from build123d import *

# Parameters (mm, degrees)
SKETCH1_W           = 38.1
SKETCH1_H           = 19.05
BOSS_EXTRUDE1_DEPTH = 12.7


with BuildPart() as part:
    # Sketch1 → Boss-Extrude1 (new body)
    with BuildSketch(Plane.XY):
        Rectangle(SKETCH1_W, SKETCH1_H)
    extrude(amount=BOSS_EXTRUDE1_DEPTH)

    # Sketch2 → Revolve1 (revolve)
    with BuildSketch(Plane(origin=(0, 0, 0), x_dir=(0, 0, -1), z_dir=(1, 0, 0))):
        Polygon((0, 0), (-800, 647.827226556), (-800, 0), align=None)
    revolve(axis=Axis((0, 0, 800), (0, 0, -1)))


solid = part.part
The model under review builds one solid part; all positions refer to its coordinate system, in mm. Give positions to 0.01 mm unless a question says otherwise; leave off trailing zeros. Loops run counter-clockwise (first coordinate to the right, second up) from the corner with the lowest first, then second, coordinate; pieces in that order, holes last. Notation, with made-up numbers: (-19.75, -38) -> (8.25, -38) arc R16 cw to (8.25, -11) -> close; hole circle Ø3 at (15.5, 22). An arc over 180 degrees is marked (long way). Answer as a JSON object with one key per item and string values. Group by question number.
Q1. Insertion check: pin 1 (1 mm diameter, centred on y = 50, z = 383, fed in from -X); pin 2 (2 mm diameter, centred on x = -401.5, z = 575.5, fed in from -Y); pin 3 (4 mm diameter, centred on y = 349, z = 692.5, fed in from -X). Each pin has a flat end and moves straight along its axis. Give the tip position at first contact, or say it passes through.
Q2. Take a section at B-B (z = 478). Write out the cut boundary in (x, y).
Q3. Wall thickness on line 1 along Y through (x, z) = (173, 371.5); line 2 along X through (y, z) = (-320, 680); line 3 along X through (y, z) = (7.5, 402.5): over which ranges is each line inside the solid? List them lowest first.
Q4. Take a section at A-A (z = 87). Write out the cut boundary in (x, y), plus the area to 3 significant figures.
Answer below:
{
 "1": {"pin 1": "stops at x = -306.51", "pin 2": "stops at y = -238.92", "pin 3": "stops at x = -441.54"},
 "2": {"outline": "circle Ø774.15 at (0, 0)"},
 "3": {"line 1": "y = -246.11 to 246.11", "line 2": "x = -448.13 to 448.13", "line 3": "x = -325.85 to 325.85"},
 "4": {"outline": "circle Ø140.9 at (0, 0)", "area": "15,600 mm2"}
}
